from build123d import *

# Parameters (mm, degrees)
SKETCH1_R           = 1.44
SKETCH1_R_2         = 1
BOSS_EXTRUDE1_DEPTH = 2


with BuildPart() as part:
    # Sketch1 → Boss-Extrude1 (new body)
    with BuildSketch(Plane(origin=(0, 0, 0), x_dir=(1, 0, 0), z_dir=(0, 1, 0))):
        Polygon((-17.332807681, 117.69771489), (-17.332807681, -38.346866508), (-6.997005855, -57.284094596), (4.918028523, -57.284094596), (15.167192319, -38.486712582), (15.167192319, 187.692065716), (10.237192319, 187.692065716), (10.237192319, 175.692065716), (-12.402807681, 175.692065716), (-12.402807681, 187.692065716), (-17.332807681, 187.692065716), align=None)
        with Locations((-13.842807681, -34.799722329)):
            Circle(SKETCH1_R, mode=Mode.SUBTRACT)
        with Locations((-1.042807681, -54.059722329)):
            Circle(SKETCH1_R, mode=Mode.SUBTRACT)
        Polygon((-2.842807681, -50.284094596), (-10.225590468, -36.757379986), (8.137192319, -36.757379986), (0.761829434, -50.284094596), align=None, mode=Mode.SUBTRACT)
        Polygon((8.167192319, -29.757379986), (-10.332807681, -29.757379986), (-10.332807681, -11.546628322), align=None, mode=Mode.SUBTRACT)
        Polygon((8.167192319, -19.934969699), (-10.332807681, -1.724218034), (8.167192319, 17.069624543), align=None, mode=Mode.SUBTRACT)
        with Locations((11.757192319, -34.799722329)):
            Circle(SKETCH1_R, mode=Mode.SUBTRACT)
        Polygon((8.167192319, 27.048047931), (-10.332807681, 8.254205353), (-10.332807681, 45.258799595), align=None, mode=Mode.SUBTRACT)
        Polygon((8.167192319, 36.870458218), (-10.332807681, 55.081209882), (8.167192319, 73.87505246), align=None, mode=Mode.SUBTRACT)
        Polygon((8.167192319, 83.853475847), (-10.332807681, 65.05963327), (-10.332807681, 102.064227512), align=None, mode=Mode.SUBTRACT)
        with Locations((-14.867807681, 183.496000094)):
            Circle(SKETCH1_R_2, mode=Mode.SUBTRACT)
        Polygon((8.167192319, 140.658903764), (-10.361742255, 121.835667033), (-10.361742255, 158.89813761), align=None, mode=Mode.SUBTRACT)
        Polygon((8.167192319, 150.481314052), (-10.332807681, 168.692065716), (8.167192319, 168.692065716), align=None, mode=Mode.SUBTRACT)
        Polygon((8.167192319, 93.675886135), (-10.332807681, 111.886637799), (8.167192319, 130.680480377), align=None, mode=Mode.SUBTRACT)
        with Locations((12.702192319, 183.496000094)):
            Circle(SKETCH1_R_2, mode=Mode.SUBTRACT)
    extrude(amount=BOSS_EXTRUDE1_DEPTH)


solid = part.part
Work out the finished part from the listing and answer in its coordinate system (mm). A direction names the side the tool comes from. Round coordinates to 2 decimals unless told otherwise and drop trailing zeros. Order: outer loops, then holes, each group sorted by start corner. A loop starts at its lowest first (then second) coordinate and runs counter-clockwise, first axis right, second up. Notation, with made-up numbers: M 41,60.5 L 85,60.5 A20 ccw 85,87.5 Z; hole C 41.5,-4.5 d11. An arc over 180 degrees is marked long. Put each result on its own line as item: value. Start each with the question number.
Q1. Section C-C, the plane z = -161 is taken. Write down the section's boundary in (x, y).
Q2. Section A-A, the plane z = -79 is taken. Write down the section's boundary in (x, y).
Q3. Section B-B, the plane z = 16 is taken. Write down the section's boundary in (x, y).
Q4. Straight lines are drawn through the part: L1, parallel to X at y = 1.3, z = -127; L2, parallel to X at y = 0.75, z = -41.5; L3, parallel to Z at x = -15, y = 0.8. For each, find the intervals that lie inside material, in ascending order. Write a range as [from, to].
Q5. A tool of negligible diameter and unlimited length cuts with its end or side. For faces 4 (the flat face through (-1, 2, -67)), 5 (the flat face through (-6.48, 0.99, 43.62)), from which of +Z, -Z, +X, -X, +Y, -Y can it reach the whole face along a straight path? Write none if from no direction.
Q6. Section D-D, the plane y = 1.7 is taken. Give the number of separate pieces and of enclosed holes in the cut face, and give its area (3 significant figures).
Q7. Flat-ended cylindrical pins translate along their axes: pin 1 (1.2 mm diameter, centred on x = -14.87, z = -183.5, fed in from -Y); pin 2 (0.6 mm diameter, centred on x = -6.5, y = 1, fed in from -Z). Find the tip coordinate at first contact, or state that the pin passes through.
Q8. For a pull along Z with two mould halves and no side action, classify faces 1 (the flat face through (9.97, 0.99, 48.02)), 2 (the flat face through (-1, 0, -67)), 3 (the flat face through (-1.23, 0.99, -149.91)) as pulls with the +Z half, pulls with the -Z half, needs draft (parallel to the pull), parting line crosses it, or undercut.
Findings below:
1. outline: M -17.33,0 L -2.52,0 L -2.52,2 L -17.33,2 Z; M 8.17,0 L 15.17,0 L 15.17,2 L 8.17,2 Z
2. outline: M -17.33,0 L -10.33,0 L -10.33,2 L -17.33,2 Z; M 3.39,0 L 15.17,0 L 15.17,2 L 3.39,2 Z
3. outline: M -17.33,0 L -10.33,0 L -10.33,2 L -17.33,2 Z; M -5.81,0 L 4.17,0 L 4.17,2 L -5.81,2 Z; M 8.17,0 L 15.17,0 L 15.17,2 L 8.17,2 Z
4. L1: x = [-17.33, -10.36], [-5.28, 4.54], [8.17, 15.17]
4. L2: x = [-17.33, -10.33], [-6.51, 3.46], [8.17, 15.17]
4. L3: z = [-187.69, -184.49], [-182.5, 33.94], [35.66, 42.62]
5. face 4: +Z, -Z, +X, -X, +Y
5. face 5: +Y, -Y
6. separate pieces: 1
6. enclosed holes: 14
6. area: 4,930 mm^2
7. pin 1: passes through
7. pin 2: stops at z = -175.69
8. face 1: pulls with the +Z half
8. face 2: needs draft
8. face 3: undercut
